Here's how the part is built. I have some questions about the finished solid (model axes, mm). A direction names the side the tool comes from. Round coordinates to 2 decimals unless told otherwise and drop trailing zeros. Loops run counter-clockwise (first coordinate to the right, second up) from the corner with the lowest first, then second, coordinate; pieces in that order, holes last. Notation, with made-up numbers: M 14,71 L 26,71 A19 ccw 26,85 Z; hole C -0.5,-35 d7. An arc over 180 degrees is marked long. Use a Markdown table: item, result.
```python
from build123d import *

# Parameters (mm, degrees)
SKETCH1_W               = 100
SKETCH1_H               = 50
BOSS_EXTRUDE1_DEPTH     = 2.5
SKETCH2_R               = 5
BOSS_EXTRUDE2_DEPTH     = 8.2
CUT_EXTRUDE1_DEPTH      = 113.314246648
CUT_EXTRUDE1_DEPTH_BACK = 113.314246648
SKETCH3_R               = 4.5
CUT_EXTRUDE4_DEPTH      = 113.314246648
CUT_EXTRUDE4_DEPTH_BACK = 113.314246648
SKETCH4_R               = 1
SKETCH6_W               = 5
SKETCH6_H               = 20
BOSS_EXTRUDE3_DEPTH     = 15
FILLET1_R               = 1
CUT_EXTRUDE5_DEPTH      = 113.805141727
CUT_EXTRUDE5_DEPTH_BACK = 113.805141727
SKETCH7_R               = 2.5


with BuildPart() as part:
    # Sketch1 → Boss-Extrude1 (new body)
    with BuildSketch(Plane.XY):
        with Locations((50, -25)):
            Rectangle(SKETCH1_W, SKETCH1_H)
    extrude(amount=BOSS_EXTRUDE1_DEPTH)

    # Sketch2 → Boss-Extrude2 (add)
    with BuildSketch(Plane(origin=(0, 0, 0), x_dir=(-1, 0, 0), z_dir=(0, 0, -1))):
        with Locations(Location((-7.5, -7.5, 0), (0, 0, 180))):
            Circle(SKETCH2_R)
        with Locations(Location((-92.5, -7.5, 0), (0, 0, 180))):
            Circle(SKETCH2_R)
        with Locations(Location((-7.5, -42.5, 0), (0, 0, 180))):
            Circle(SKETCH2_R)
        with Locations(Location((-92.5, -42.5, 0), (0, 0, 180))):
            Circle(SKETCH2_R)
    extrude(amount=BOSS_EXTRUDE2_DEPTH)

    # Sketch3 → Cut-Extrude1 (cut, two sides: drawn at the far end of the back side and taken through both)
    with BuildSketch(Plane.XY.offset(2.5).offset(-CUT_EXTRUDE1_DEPTH_BACK)):
        with Locations((30, -25)):
            Circle(SKETCH3_R)
    extrude(amount=CUT_EXTRUDE1_DEPTH + CUT_EXTRUDE1_DEPTH_BACK, mode=Mode.SUBTRACT)

    # Sketch4 → Cut-Extrude4 (cut, two sides: drawn at the far end of the back side and taken through both)
    with BuildSketch(Plane(origin=(0, 0, -8.2), x_dir=(-1, 0, 0), z_dir=(0, 0, -1)).offset(-CUT_EXTRUDE4_DEPTH_BACK)):
        with Locations((-92.5, -7.5)):
            Circle(SKETCH4_R)
        with Locations((-92.5, -42.5)):
            Circle(SKETCH4_R)
        with Locations((-7.5, -42.5)):
            Circle(SKETCH4_R)
        with Locations((-7.5, -7.5)):
            Circle(SKETCH4_R)
    extrude(amount=CUT_EXTRUDE4_DEPTH + CUT_EXTRUDE4_DEPTH_BACK, mode=Mode.SUBTRACT)

    # Sketch6 → Boss-Extrude3 (add)
    with BuildSketch(Plane.XY.offset(2.5)):
        with Locations((22.1, -25)):
            Rectangle(SKETCH6_W, SKETCH6_H)
        with Locations((37.9, -25)):
            Rectangle(SKETCH6_W, SKETCH6_H)
    extrude(amount=BOSS_EXTRUDE3_DEPTH)

    # Fillet1
    fillet1_edges = [part.edges().sort_by_distance(p)[0] for p in [
        (24.6, -25, 2.5),
        (24.6, -35, 10),
        (22.1, -15, 2.5),
        (24.6, -15, 10),
        (19.6, -25, 2.5),
        (19.6, -15, 10),
        (22.1, -35, 2.5),
        (19.6, -35, 10),
        (24.6, -25, 17.5),
        (22.1, -15, 17.5),
        (19.6, -25, 17.5),
        (22.1, -35, 17.5),
        (37.9, -15, 2.5),
        (40.4, -15, 10),
        (35.4, -25, 2.5),
        (35.4, -15, 10),
        (37.9, -35, 2.5),
        (35.4, -35, 10),
        (40.4, -25, 2.5),
        (40.4, -35, 10),
        (37.9, -15, 17.5),
        (35.4, -25, 17.5),
        (37.9, -35, 17.5),
        (40.4, -25, 17.5),
    ]]
    fillet(fillet1_edges, radius=FILLET1_R)

    # Sketch7 → Cut-Extrude5 (cut, two sides: drawn at the far end of the back side and taken through both)
    with BuildSketch(Plane.XY.offset(2.5).offset(-CUT_EXTRUDE5_DEPTH_BACK)):
        with Locations((80.857536388, -25)):
            Circle(SKETCH7_R)
    extrude(amount=CUT_EXTRUDE5_DEPTH + CUT_EXTRUDE5_DEPTH_BACK, mode=Mode.SUBTRACT)


solid = part.part
```
Q1. We'd pull the mould along Y, two halves only. Please class faces 1 (the cylindrical face through (12.27, -9, -4.04)), 2 (the flat face through (22, -35, 10)), 3 (the flat face through (19.6, -25, 10)): pulls with the +Y half, pulls with the -Y half, needs draft (parallel to the pull), parting line crosses it, or undercut.
Return value:
| item | result |
|---|---|
| face 1 | undercut |
| face 2 | pulls with the -Y half |
| face 3 | needs draft |
Q2. Imagine slicing it at C-C, the plane z = 9. Please give me the cut outline in (x, y).
Return value:
| item | result |
|---|---|
| outline | M 19.6,-34 A1 ccw 20.6,-35 L 23.6,-35 A1 ccw 24.6,-34 L 24.6,-16 A1 ccw 23.6,-15 L 20.6,-15 A1 ccw 19.6,-16 Z; M 35.4,-34 A1 ccw 36.4,-35 L 39.4,-35 A1 ccw 40.4,-34 L 40.4,-16 A1 ccw 39.4,-15 L 36.4,-15 A1 ccw 35.4,-16 Z |
Q3. Imagine slicing it at D-D, the plane x = 30. Please give me the cut outline in (y, z).
Return value:
| item | result |
|---|---|
| outline | M -50,0 L -29.5,0 L -29.5,2.5 L -50,2.5 Z; M -20.5,0 L 0,0 L 0,2.5 L -20.5,2.5 Z |
Q4. Will these pins go through, and if not, where does the flat tip stop? P1, Ø10.5, axis at y = -27, z = 12.5, coming from the -X side; P2, Ø1, axis at x = 15.5, y = -18, coming from the +Z side; P3, Ø0.9, axis at x = 38, z = 8, coming from the +Y side.
Return value:
| item | result |
|---|---|
| P1 | stops at x = 19.6 |
| P2 | stops at z = 2.5 |
| P3 | stops at y = -15 |
Q5. I need wall thicknesses on line 1 (Y direction, x = 7.5, z = -0.25); line 2 (Y direction, x = 30, z = 0.9); line 3 (X direction, y = -8, z = -3.75). Which ranges of each line are inside material? Lowest first, please. Write a range as from..to.
Return value:
| item | result |
|---|---|
| line 1 | y = -47.5..-43.5, -41.5..-37.5, -12.5..-8.5, -6.5..-2.5 |
| line 2 | y = -50..-29.5, -20.5..0 |
| line 3 | x = 2.53..6.63, 8.37..12.47, 87.53..91.63, 93.37..97.47 |
Q6. Imagine slicing it at B-B, the plane y = -42.5. Please give me the cut outline in (x, z).
Return value:
| item | result |
|---|---|
| outline | M 0,0 L 2.5,0 L 2.5,-8.2 L 6.5,-8.2 L 6.5,2.5 L 0,2.5 Z; M 8.5,-8.2 L 12.5,-8.2 L 12.5,0 L 87.5,0 L 87.5,-8.2 L 91.5,-8.2 L 91.5,2.5 L 8.5,2.5 Z; M 93.5,-8.2 L 97.5,-8.2 L 97.5,0 L 100,0 L 100,2.5 L 93.5,2.5 Z |
Q7. For faces 4 (the flat face through (22, -15, 10)), 5 (the flat face through (40.4, -25, 10)), 6 (the flat face through (38, -35, 10)), 7 (the flat face through (49, -25, 0)), 8 (the flat face through (35.4, -25, 10)), which set-ups out of +Z, -Z, +X, -X, +Y, -Y let a thin tool reach every point of the face, with its end or its side?
Return value:
| item | result |
|---|---|
| face 4 | +Z, +X, -X, +Y |
| face 5 | +Z, +X, +Y, -Y |
| face 6 | +Z, +X, -X, -Y |
| face 7 | -Z |
| face 8 | +Z, +Y, -Y |
Q8. Imagine slicing it at A-A, the plane x = 92.5. Please give me the cut outline in (y, z), then the cut area to 3 significant figures.
Return value:
| item | result |
|---|---|
| outline | M -50,0 L -47.5,0 L -47.5,-8.2 L -43.5,-8.2 L -43.5,2.5 L -50,2.5 Z; M -41.5,-8.2 L -37.5,-8.2 L -37.5,0 L -12.5,0 L -12.5,-8.2 L -8.5,-8.2 L -8.5,2.5 L -41.5,2.5 Z; M -6.5,-8.2 L -2.5,-8.2 L -2.5,0 L 0,0 L 0,2.5 L -6.5,2.5 Z |
| area | 246 mm^2 |
